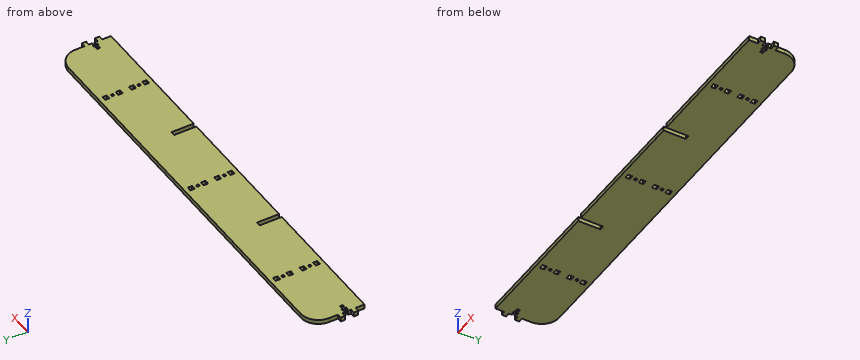
```python
from build123d import *

# Parameters (mm, degrees)
ESQUISSE1_R        = 1.5
ESQUISSE1_W        = 5
ESQUISSE1_H        = 5
BOSS_EXTRU_1_DEPTH = 5
CONG_1_R           = 20


with BuildPart() as part:
    # Esquisse1 → Boss.-Extru.1 (new body)
    with BuildSketch(Plane.XY):
        Polygon((0, 21.5), (0, 25), (-5, 25), (-5, 30), (0, 30), (0, 60), (475, 60), (475, 30), (480, 30), (480, 25), (475, 25), (475, 21.5), (472, 21.5), (472, 22.6), (469.7, 22.6), (469.7, 21.5), (465, 21.5), (465, 18.5), (469.7, 18.5), (469.7, 17.4), (472, 17.4), (472, 18.5), (475, 18.5), (475, 15), (480, 15), (480, 10), (475, 10), (475, 0), (320, 0), (320, 25), (315, 25), (315, 0), (160, 0), (160, 25), (155, 25), (155, 0), (0, 0), (0, 10), (-5, 10), (-5, 15), (0, 15), (0, 18.5), (3, 18.5), (3, 17.4), (5.3, 17.4), (5.3, 18.5), (10, 18.5), (10, 21.5), (5.3, 21.5), (5.3, 22.6), (3, 22.6), (3, 21.5), align=None)
        with Locations((397.5, 15)):
            Circle(ESQUISSE1_R, mode=Mode.SUBTRACT)
        with Locations((397.5, 45)):
            Circle(ESQUISSE1_R, mode=Mode.SUBTRACT)
        with Locations((237.5, 15)):
            Circle(ESQUISSE1_R, mode=Mode.SUBTRACT)
        with Locations((237.5, 45)):
            Circle(ESQUISSE1_R, mode=Mode.SUBTRACT)
        with Locations((77.5, 15)):
            Circle(ESQUISSE1_R, mode=Mode.SUBTRACT)
        with Locations((77.5, 45)):
            Circle(ESQUISSE1_R, mode=Mode.SUBTRACT)
        with Locations((397.5, 7.5)):
            Rectangle(ESQUISSE1_W, ESQUISSE1_H, mode=Mode.SUBTRACT)
        with Locations((397.5, 22.5)):
            Rectangle(ESQUISSE1_W, ESQUISSE1_H, mode=Mode.SUBTRACT)
        with Locations((397.5, 37.5)):
            Rectangle(ESQUISSE1_W, ESQUISSE1_H, mode=Mode.SUBTRACT)
        with Locations((397.5, 52.5)):
            Rectangle(ESQUISSE1_W, ESQUISSE1_H, mode=Mode.SUBTRACT)
        with Locations((237.5, 7.5)):
            Rectangle(ESQUISSE1_W, ESQUISSE1_H, mode=Mode.SUBTRACT)
        with Locations((237.5, 22.5)):
            Rectangle(ESQUISSE1_W, ESQUISSE1_H, mode=Mode.SUBTRACT)
        with Locations((237.5, 37.5)):
            Rectangle(ESQUISSE1_W, ESQUISSE1_H, mode=Mode.SUBTRACT)
        with Locations((237.5, 52.5)):
            Rectangle(ESQUISSE1_W, ESQUISSE1_H, mode=Mode.SUBTRACT)
        with Locations((77.5, 7.5)):
            Rectangle(ESQUISSE1_W, ESQUISSE1_H, mode=Mode.SUBTRACT)
        with Locations((77.5, 22.5)):
            Rectangle(ESQUISSE1_W, ESQUISSE1_H, mode=Mode.SUBTRACT)
        with Locations((77.5, 37.5)):
            Rectangle(ESQUISSE1_W, ESQUISSE1_H, mode=Mode.SUBTRACT)
        with Locations((77.5, 52.5)):
            Rectangle(ESQUISSE1_W, ESQUISSE1_H, mode=Mode.SUBTRACT)
    extrude(amount=BOSS_EXTRU_1_DEPTH)

    # Congé1
    cong_1_edges = [part.edges().sort_by_distance(p)[0] for p in [
        (0, 60, 2.5),
        (475, 60, 2.5),
    ]]
    fillet(cong_1_edges, radius=CONG_1_R)


solid = part.part
```
For this review, take the finished solid that the model builds, in its own axes (mm). Give positions to 0.01 mm unless a question says otherwise; leave off trailing zeros. Answer as a JSON object with one key per item and string values. Group by question number.
Item 1: For pin 1 Ø0.9 at (y, z) = (22, 2) entering from -X; pin 2 Ø0.9 at (y, z) = (19.5, 3) entering from +X; pin 3 Ø1.5 at (x, z) = (157.5, 1.5) entering from -Y, all flat-tipped, find the tip position at first contact; note any pin that passes through.
Item 2: For probe 1 along X at (y, z) = (8, 0.65); probe 2 along Y at (x, z) = (399.5, 4.15); probe 3 along X at (y, z) = (38.5, 3), list the stretches that pass through material, from the lowest coordinate up. Write a range as [from, to].
Item 3: Consider section A-A on z = 2.45. Count the separate pieces of the cut face and the enclosed holes in it, plus the area to 3 significant figures.
Check result:
{
 "1": {"pin 1": "stops at x = 0", "pin 2": "stops at x = 465", "pin 3": "stops at y = 25"},
 "2": {"probe 1": "x = [0, 75], [80, 155], [160, 235], [240, 315], [320, 395], [400, 475]", "probe 2": "y = [0, 5], [10, 20], [25, 35], [40, 50], [55, 60]", "probe 3": "x = [0, 75], [80, 235], [240, 395], [400, 475]"},
 "3": {"separate pieces": "1", "enclosed holes": "18", "area": "27,800 mm^2"}
}
